Check sheet for the modelled part. Datum: model origin and axes. Units: mm. Give positions to 0.01 mm unless a question says otherwise; leave off trailing zeros. Order: outer loops, then holes, each group sorted by start corner. A loop starts at its lowest first (then second) coordinate and runs counter-clockwise, first axis right, second up. Notation, with made-up numbers: (87.25, -15) -> (130.25, -15) arc R15 ccw to (130.25, -2) -> close; hole circle Ø4 at (26.25, 75). An arc over 180 degrees is marked (long way). Answer in a Markdown table with one row per item. Add a question column.
(1) Cross-section at A-A (x = -14.5). Record the cut outline in (y, z) (3 decimals), then the cut area to 3 significant figures.
(2) Release check for a two-part mould opening along X. For faces 1 (the face through (-26.281, 2, -15)), 2 (the face through (-14, 2, -56.216)), 3 (the face through (-11.598, 1.61, 5.848)), 4 (the face through (-0.881, 2, -15)) record: released by +X, released by -X, zero draft, split by the parting line, or undercut.
(3) Thickness scan on L1, parallel to X at y = 2.5, z = 7; L2, parallel to Z at x = -12, y = 1.9; L3, parallel to Z at x = -1.75, y = 2.4. Record the ranges inside material, lowest first. Write a range as [from, to].
```python
from build123d import *

# Parameters (mm, degrees)
SKETCH1_W           = 25.4
SKETCH1_H           = 81.175
BOSS_EXTRUDE1_DEPTH = 3.175
SKETCH2_R           = 2
CUT_EXTRUDE1_DEPTH  = 63.137257853
FILLET1_R           = 2.54


with BuildPart() as part:
    # Sketch1 → Boss-Extrude1 (new body)
    with BuildSketch(Plane(origin=(0, 0, 0), x_dir=(1, 0, 0), z_dir=(0, 1, 0))):
        with Locations((-13.581081081, 15.628716216)):
            Rectangle(SKETCH1_W, SKETCH1_H)
    extrude(amount=BOSS_EXTRUDE1_DEPTH)

    # Sketch2 → Cut-Extrude1 (cut, through all)
    with BuildSketch(Plane(origin=(0, 3.175, 0), x_dir=(1, 0, 0), z_dir=(0, 1, 0))):
        with Locations(Location((-13.581081081, -6.108783784, 0), (0, 0, 270))):
            Circle(SKETCH2_R)
    extrude(amount=-CUT_EXTRUDE1_DEPTH, mode=Mode.SUBTRACT)

    # Fillet1
    fillet1_edges = [part.edges().sort_by_distance(p)[0] for p in [
        (-26.281081081, 1.5875, -56.216216216),
        (-0.881081081, 1.5875, -56.216216216),
        (-0.881081081, 1.5875, 24.958783784),
        (-26.281081081, 1.5875, 24.958783784),
    ]]
    fillet(fillet1_edges, radius=FILLET1_R)


solid = part.part
```
Answer below:
| question | item | result |
|---|---|---|
| 1 | outline | (0, -56.216) -> (3.175, -56.216) -> (3.175, 4.332) -> (0, 4.332) -> close; (0, 7.885) -> (3.175, 7.885) -> (3.175, 24.959) -> (0, 24.959) -> close |
| 1 | area | 246 mm² |
| 2 | face 1 | released by -X |
| 2 | face 2 | zero draft |
| 2 | face 3 | undercut |
| 2 | face 4 | released by +X |
| 3 | L1 | x = [-26.28, -15.37], [-11.79, -0.88] |
| 3 | L2 | z = [-56.22, 4.88], [7.33, 24.96] |
| 3 | L3 | z = [-55.59, 24.33] |
